```python
from build123d import *

# Parameters (mm, degrees)
F0_W     = 200
F0_H     = 150
F1_DEPTH = 9
F2_W     = 10
F2_H     = 12.5
F3_DEPTH = 25
F4_R     = 5


with BuildPart() as f1:
    # F0 (on Top) → F1 (new body)
    with BuildSketch(Plane.XY):
        Rectangle(F0_W, F0_H)
    extrude(amount=F1_DEPTH)

    # F2 (on face) → F3 (cut)
    with BuildSketch(Plane.XY.offset(9)):
        Polygon((87.4994372893, -64.5627596692), (87.4994372893, 60.4372403308), (-87.5005627107, 60.4372403308), (-87.5005627107, 34.7239444211), (-41.0005627107, 34.7239444211), (-33.5005627107, 34.7239444211), (-33.5005627107, 26.7239444211), (-38.5005627107, 26.7239444211), (-38.5005627107, 29.7239444211), (-46.0005627107, 29.7239444211), (-87.5005627107, 29.7239444211), (-87.5005627107, 2.7372403308), (-92.5005627107, -0.2627596692), (-100, -0.2627596692), (-100, -3.8627596692), (-92.5005627107, -3.8627596692), (-87.5005627107, -6.8627596692), (-87.5005627107, -33.2760555789), (-38.5005627107, -33.2760555789), (-38.5005627107, -30.2760555789), (-33.5005627107, -30.2760555789), (-33.5005627107, -38.2760555789), (-41.0005627107, -38.2760555789), (-46.0005627107, -38.2760555789), (-87.5005627107, -38.2760555789), (-87.5005627107, -64.5627596692), (-77.5005627107, -64.5627596692), align=None)
        with BuildLine():
            Line((-77.3623862099, 50.4372403308), (-74.3623862099, 50.4372403308))
            Line((-74.3623862099, 50.4372403308), (60.6376137901, 50.4372403308))
            Line((60.6376137901, 50.4372403308), (74.4994372893, 50.4372403308))
            Line((74.4994372893, 50.4372403308), (77.4994372893, 50.4372403308))
            Line((77.4994372893, 50.4372403308), (77.4994372893, 47.4372403308))
            Line((77.4994372893, 47.4372403308), (77.4994372893, -54.5627596692))
            Line((77.4994372893, -54.5627596692), (60.6376137901, -54.5627596692))
            Line((60.6376137901, -54.5627596692), (-77.5005627107, -54.5627596692))
            Line((-77.5005627107, -54.5627596692), (-77.5005627107, -51.5627596692))
            Line((-77.5005627107, -51.5627596692), (60.6376137901, -51.5627596692))
            Line((60.6376137901, -51.5627596692), (69.4994372893, -51.5627596692))
            ThreePointArc((69.4994372893, -51.5627596692), (73.0349711952, -50.0982935751), (74.4994372893, -46.5627596692))
            Line((74.4994372893, -46.5627596692), (74.4994372893, 42.4372403308))
            ThreePointArc((74.4994372893, 42.4372403308), (73.0349711952, 45.9727742368), (69.4994372893, 47.4372403308))
            Line((69.4994372893, 47.4372403308), (60.6376137901, 47.4372403308))
            Line((60.6376137901, 47.4372403308), (57.6376137901, 47.4372403308))
            Line((57.6376137901, 47.4372403308), (-74.3623862099, 47.4372403308))
            Line((-74.3623862099, 47.4372403308), (-77.3623862099, 47.4372403308))
            Line((-77.3623862099, 47.4372403308), (-77.3623862099, 50.4372403308))
        make_face(mode=Mode.SUBTRACT)
        Polygon((39.9994372893, -27.0627596692), (39.9994372893, -2.0627596692), (39.9994372893, 22.9372403308), (39.9994372893, 35.4372403308), (49.9994372893, 35.4372403308), (49.9994372893, 22.9372403308), (49.9994372893, -27.0627596692), (49.9994372893, -39.5627596692), (39.9994372893, -39.5627596692), align=None, mode=Mode.SUBTRACT)
        Polygon((39.9994372893, 22.9372403308), (39.9994372893, -2.0627596692), (39.9994372893, -27.0627596692), (49.9994372893, -27.0627596692), (49.9994372893, 22.9372403308), align=None)
        with Locations((44.9994372893, 29.1872403308)):
            Rectangle(F2_W, F2_H)
        with Locations((44.9994372893, -33.3127596692)):
            Rectangle(F2_W, F2_H)
        Polygon((-87.5005627107, 60.4372403308), (87.4994372893, 60.4372403308), (87.4994372893, -64.5627596692), (-77.5005627107, -64.5627596692), (-87.5005627107, -64.5627596692), (-87.5005627107, -38.2760555789), (-46.0005627107, -38.2760555789), (-41.0005627107, -38.2760555789), (-33.5005627107, -38.2760555789), (-33.5005627107, -30.2760555789), (-38.5005627107, -30.2760555789), (-38.5005627107, -33.2760555789), (-87.5005627107, -33.2760555789), (-87.5005627107, -6.8627596692), (-92.5005627107, -3.8627596692), (-100, -3.8627596692), (-100, -75), (100, -75), (100, 75), (-100, 75), (-100, -0.2627596692), (-92.5005627107, -0.2627596692), (-87.5005627107, 2.7372403308), (-87.5005627107, 29.7239444211), (-46.0005627107, 29.7239444211), (-38.5005627107, 29.7239444211), (-38.5005627107, 26.7239444211), (-33.5005627107, 26.7239444211), (-33.5005627107, 34.7239444211), (-41.0005627107, 34.7239444211), (-87.5005627107, 34.7239444211), align=None)
    extrude(amount=-F3_DEPTH, mode=Mode.SUBTRACT)

    # F4
    f4_edges = [f1.edges().sort_by_distance(p)[0] for p in [
        (77.499437, 50.43724, 4.5),
        (77.499437, -54.56276, 4.5),
    ]]
    fillet(f4_edges, radius=F4_R)


solid = f1.part
```
Build history of the part. All positions in model axes, mm. A direction names the side the tool comes from. Coordinates: 2 decimals unless noted, no trailing zeros. Write each loop counter-clockwise with the first axis right and the second up, starting at its lowest first coordinate (ties: lowest second). Pieces come first, ordered by that corner, then holes.
1. Band-saw the part on B-B, the plane z = 4.5. Give the cut face in (x, y).
Answer block:
outline: (-77.5, -54.56) - (72.5, -54.56) arc R5 ccw to (77.5, -49.56) - (77.5, 45.44) arc R5 ccw to (72.5, 50.44) - (-77.36, 50.44) - (-77.36, 47.44) - (69.5, 47.44) arc R5 cw to (74.5, 42.44) - (74.5, -46.56) arc R5 cw to (69.5, -51.56) - (-77.5, -51.56) - close
2. Drill centre lines: probe 1 along Y at (x, z) = (29.5, 1.5); probe 2 along X at (y, z) = (-46, 7.75); probe 3 along X at (y, z) = (43.5, 7.75). Where is each one in solid material? Low to high.
Answer block:
probe 1: y = -54.56 to -51.56, 47.44 to 50.44
probe 2: x = 74.5 to 77.5
probe 3: x = 74.39 to 77.5
3. Band-saw the part on A-A, the plane x = 65. Give the cut face in (y, z).
Answer block:
outline: (-54.56, 0) - (-51.56, 0) - (-51.56, 9) - (-54.56, 9) - close; (47.44, 0) - (50.44, 0) - (50.44, 9) - (47.44, 9) - close
4. Drop flat-ended pins along their axis: pin 1 (4.5 mm diameter, centred on y = -17, z = 4.5, fed in from -X); pin 2 (1.5 mm diameter, centred on y = 49.5, z = 3, fed in from -X). Give the stop position or say it passes through.
Answer block:
pin 1: stops at x = 74.5
pin 2: stops at x = -77.36
5. Band-saw the part on C-C, the plane y = 20. Give the cut face in (x, z).
Answer block:
outline: (74.5, 0) - (77.5, 0) - (77.5, 9) - (74.5, 9) - close
6. 3-axis set-ups, long thin cutter, end or side, ignore diameter. For faces 5 (the flat face through (-5, -51.563, 5)), 6 (the flat face through (0, 49, 0)), 7 (the flat face through (-77.362, 49, 5)): which of +Z, -Z, +X, -X, +Y, -Y reach the whole face in a straight line?
Answer block:
face 5: +Z, -Z, -X
face 6: -Z, +X, -X, +Y, -Y
face 7: +Z, -Z, -X, +Y
7. Pull direction Y, two halves, no side cores. Call faces 1 (the flat face through (-77.501, -53, 5)), 2 (the cylindrical face through (76.074, -53.059, 4.437)), 3 (the cylindrical face through (73.074, 45.934, 4.563)), 4 (the flat face through (-3, 47.437, 5)): released by +Y, released by -Y, zero draft, split by the parting line, or undercut.
Answer block:
face 1: zero draft
face 2: released by -Y
face 3: undercut
face 4: undercut
